Drawing for the job (mm, zero at the part's lowest x, y, z). A direction names the side the tool comes from. Coordinates: 2 decimals unless noted, no trailing zeros. Order: outer loops, then holes, each group sorted by start corner. A loop starts at its lowest first (then second) coordinate and runs counter-clockwise, first axis right, second up. Notation, with made-up numbers: (50, 4.5) - (109, 4.5) arc R21 cw to (109, 35.5) - close; hole circle Ø9 at (-10.5, 60). An arc over 180 degrees is marked (long way). Answer as CSV lines item,"result". Start each with the question number.
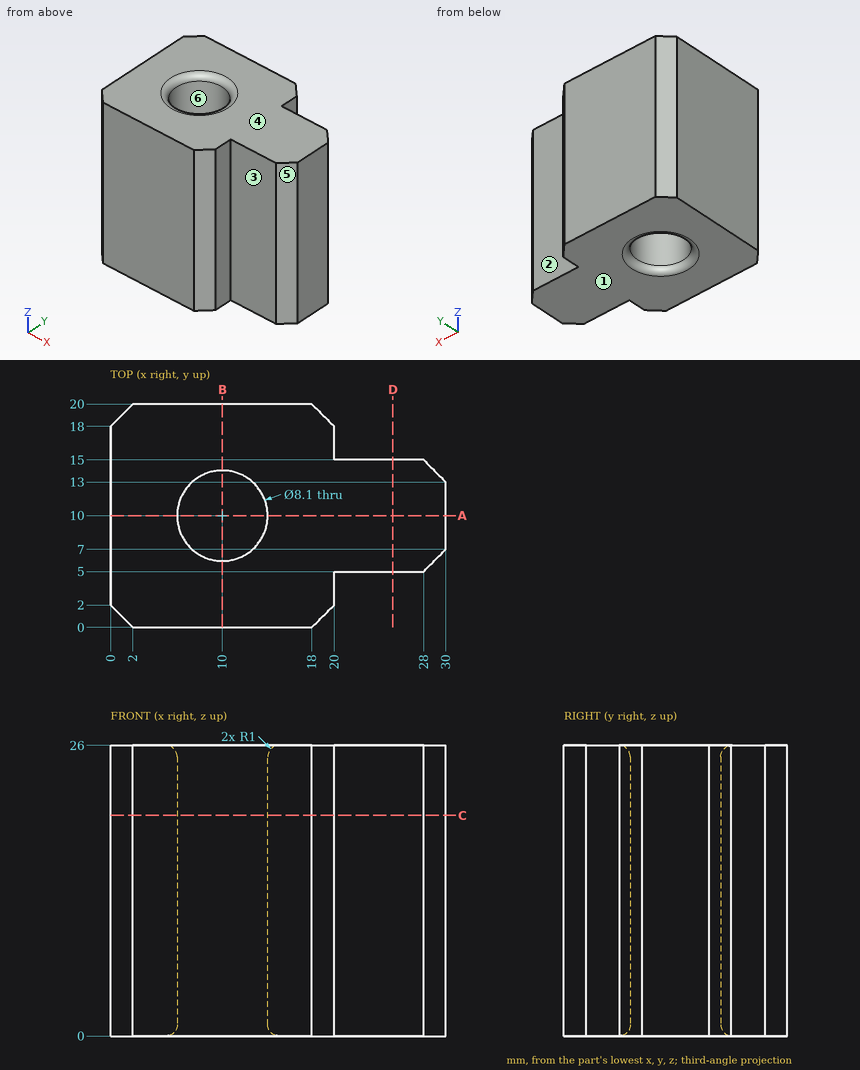
(1) Band-saw the part on B-B on x = 10. List the corners of the cut face in (y, z).
(2) Band-saw the part on D-D on x = 25.25. List the corners of the cut face in (y, z).
(3) Probe L1, parallel to Y at x = 10, z = 17.5; L2, parallel to X at y = 3, z = 4.25; L3, parallel to Y at x = 8, z = 18.5. List the from-to ranges inside material, lowest first. Write a range as [from, to].
(4) Band-saw the part on C-C on z = 19.75. List the corners of the cut face in (x, y).
(5) Pull direction Y, two halves, no side cores. Call the marked faces 4, 5 and 6: +Y half, -Y half, draft (parallel to the pull), parting line (faces both ways), or undercut.
(6) Drop flat-ended pins along their axis: pin 1 Ø6 at (y, z) = (5, 4.5) entering from +X; pin 2 Ø3.5 at (y, z) = (16, 18.5) entering from +X; pin 3 Ø2.5 at (x, z) = (24.5, 11.5) entering from -Y; pin 4 Ø7.5 at (x, y) = (10, 10) entering from +Z. Give the stop position or say it passes through.
(7) Band-saw the part on A-A on y = 10. List the corners of the cut face in (x, z), plus the area to 3 significant figures.
(8) Which spindle directions (+Z, -Z, +X, -X, +Y, -Y) get a long thin tool onto all of the face, cutting with end or side? Do the marked faces 1, 2 and 3. Say none if no direction does.
Filled in:
1,outline,"(0, 0) - (4.95, 0) arc R1 ccw to (5.95, 1) - (5.95, 25) arc R1 ccw to (4.95, 26) - (0, 26) - close; (14.05, 1) arc R1 ccw to (15.05, 0) - (20, 0) - (20, 26) - (15.05, 26) arc R1 ccw to (14.05, 25) - close"
2,outline,"(5, 0) - (15, 0) - (15, 26) - (5, 26) - close"
3,L1,"y = [0, 5.95], [14.05, 20]"
3,L2,"x = [0, 20]"
3,L3,"y = [0, 6.48], [13.52, 20]"
4,outline,"(0, 2) - (2, 0) - (18, 0) - (20, 2) - (20, 5) - (28, 5) - (30, 7) - (30, 13) - (28, 15) - (20, 15) - (20, 18) - (18, 20) - (2, 20) - (0, 18) - close; hole circle Ø8.1 at (10, 10)"
5,face 4,"draft"
5,face 5,"-Y half"
5,face 6,"undercut"
6,pin 1,"stops at x = 30"
6,pin 2,"stops at x = 28.75"
6,pin 3,"stops at y = 5"
6,pin 4,"passes through"
7,outline,"(0, 0) - (4.95, 0) arc R1 ccw to (5.95, 1) - (5.95, 25) arc R1 ccw to (4.95, 26) - (0, 26) - close; (14.05, 1) arc R1 ccw to (15.05, 0) - (30, 0) - (30, 26) - (15.05, 26) arc R1 ccw to (14.05, 25) - close"
7,area,"569 mm^2"
8,face 1,"-Z, +X, -X, +Y, -Y"
8,face 2,"+Z, -Z, +X, +Y"
8,face 3,"+Z, -Z, +X, -Y"
